```python
from build123d import *

# Parameters (mm, degrees)
F1_DEPTH      = 25.4
F3_T          = -3.175
F2_R          = 7.62
F4_DEPTH      = 22.86
F4_DEPTH_BACK = 22.225
F5_R          = 1.1967045105
F6_DEPTH      = 7.62
F7_R          = 0.0635
F8_DEPTH      = 12.7


# Not quite as in the source:
# - a feature names something its author has since deleted; it is built from what else it names


with BuildPart() as f1:
    # F0 (on Top) → F1 (new body)
    with BuildSketch(Plane.XY):
        Polygon((-38.1, 7.0371161437), (-38.1, -7.0371161437), (0, -19.05), (127, -19.05), (127, 19.05), (0, 19.05), align=None)
    extrude(amount=F1_DEPTH)

    # F3
    f3_openings = [f1.faces().sort_by_distance(p)[0] for p in [
        (49.931192, 0, 25.4),
    ]]
    offset(amount=F3_T, openings=f3_openings)

    # F2 (on face) → F4 (join, two sides)
    with BuildSketch(Plane.XY.offset(25.4)) as f4_sk:
        Circle(F2_R)
        with Locations((38.1, 0)):
            Circle(F2_R)
        with Locations((76.2, 0)):
            Circle(F2_R)
        with Locations((114.3, 0)):
            Circle(F2_R)
    extrude(amount=F4_DEPTH)
    extrude(f4_sk.sketch, amount=-F4_DEPTH_BACK)

    # F5 (on face) → F6 (cut)
    with BuildSketch(Plane.XY.offset(25.4)):
        with Locations((1.6406770326, 17.5694916397)):
            Circle(F5_R)
        with Locations((62.6006770326, 17.5694916397)):
            Circle(F5_R)
        with Locations((123.5606770326, 17.5694916397)):
            Circle(F5_R)
        with Locations((-36.748547107, 0)):
            Circle(F5_R)
        with Locations((62.6006770326, -17.4930030425)):
            Circle(F5_R)
        with Locations((123.5606770326, -17.4930030425)):
            Circle(F5_R)
        with Locations((1.6406770326, -17.4930030425)):
            Circle(F5_R)
    extrude(amount=-F6_DEPTH, mode=Mode.SUBTRACT)

    # F7 (on face) → F8 (cut)
    with BuildSketch(Plane(origin=(-5.4633155562, -17.3274232219, 0), x_dir=(0.9537169507, -0.3007057995, 0), z_dir=(-0.3007057995, -0.9537169507, 0))):
        with Locations((-32.5760804117, 0.0889)):
            Circle(F7_R)
    extrude(amount=-F8_DEPTH, mode=Mode.SUBTRACT)


solid = f1.part
```
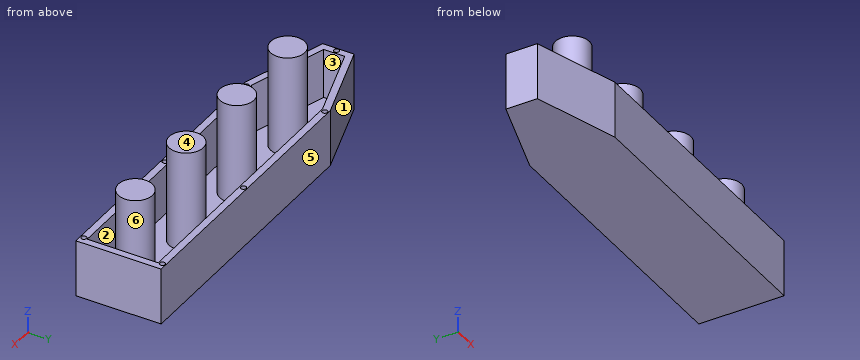
Model file for the job. Use its own axes, mm. Face numbers are marked on the shaded views. A direction names the side the tool comes from. Round coordinates to 2 decimals unless told otherwise and drop trailing zeros. Write each loop counter-clockwise with the first axis right and the second up, starting at its lowest first coordinate (ties: lowest second). Pieces come first, ordered by that corner, then holes. Notation, with made-up numbers: (83, -26) - (128, -26) arc R36 cw to (128, 12) - close; hole circle Ø5 at (58, 61). An arc over 180 degrees is marked (long way). Use CSV: the item, a comma, the result in double quotes. Start each with the question number.
Item 1: Pin check, flat tips, straight feed: P1, Ø5, axis at y = 7.5, z = 32.5, coming from the +X side; P2, Ø0.7, axis at x = -37, y = 0, coming from the +Z side; P3, Ø4, axis at x = 123.56, y = 17.57, coming from the +Z side. Stop position of each tip, or through.
Item 2: Band-saw the part on D-D (z = 40). Write the cut outline in (x, y).
Item 3: Band-saw the part on A-A (z = 11). Write the cut outline in (x, y) (3 decimals), and give its area (3 significant figures).
Item 4: Band-saw the part on B-B (x = 50). Write the cut outline in (y, z) (3 decimals).
Item 5: Drill centre lines: L1, parallel to Y at x = 91.5, z = 13 (3 decimals); L2, parallel to X at y = -3, z = 40.5; L3, parallel to X at y = -4, z = 33. Where is each one in solid material? Low to high. Write a range as [from, to].
Item 6: Tool access for the marked faces 1 and 2: list every direction of +Z, -Z, +X, -X, +Y, -Y with a clear straight run to the whole face (end or side of a thin tool).
Item 7: Two-plate mould, pull along Y, no slides. Class the marked faces 3, 4, 5 and 6: released by +Y, released by -Y, zero draft, split by the parting line, or undercut.
Item 8: Band-saw the part on C-C (y = 12). Write the cut outline in (x, z) (3 decimals), and give its area (3 significant figures).
Checked values:
1,P1,"stops at x = 120.05"
1,P2,"stops at z = 17.78"
1,P3,"stops at z = 25.4"
2,outline,"circle Ø15.24 at (0, 0); circle Ø15.24 at (38.1, 0); circle Ø15.24 at (76.2, 0); circle Ø15.24 at (114.3, 0)"
3,outline,"(-38.1, -7.037) - (0, -19.05) - (127, -19.05) - (127, 19.05) - (0, 19.05) - (-38.1, 7.037) - close; circle Ø15.24 at (0, 0); circle Ø15.24 at (38.1, 0); circle Ø15.24 at (76.2, 0); circle Ø15.24 at (114.3, 0); hole (-34.925, -4.709) - (0.489, -15.875) - (123.825, -15.875) - (123.825, 15.875) - (0.489, 15.875) - (-34.925, 4.709) - close"
3,area,"1,920 mm²"
4,outline,"(-19.05, 0) - (19.05, 0) - (19.05, 25.4) - (15.875, 25.4) - (15.875, 3.175) - (-15.875, 3.175) - (-15.875, 25.4) - (-19.05, 25.4) - close"
5,L1,"y = [-19.05, -15.875], [15.875, 19.05]"
5,L2,"x = [-7, 7], [31.1, 45.1], [69.2, 83.2], [107.3, 121.3]"
5,L3,"x = [-6.49, 6.49], [31.61, 44.59], [69.71, 82.69], [107.81, 120.79]"
6,face 1,"+Z, -Z, -X, +Y"
6,face 2,"+Z"
7,face 3,"undercut"
7,face 4,"zero draft"
7,face 5,"released by +Y"
7,face 6,"undercut"
8,outline,"(-22.36, 0) - (127, 0) - (127, 25.4) - (123.825, 25.4) - (123.825, 3.175) - (-11.801, 3.175) - (-11.801, 25.4) - (-22.36, 25.4) - close"
8,area,"779 mm²"
